Autodesk Inventor part; units mm, degrees
ref_plane "YZ Plane" through (0, 0, 0) normal (1, 0, 0) x (0, 1, 0)
ref_plane "XZ Plane" through (0, 0, 0) normal (0, 1, 0) x (-1, 0, 0)
ref_plane "XY Plane" through (0, 0, 0) normal (0, 0, 1) x (1, 0, 0)
sketch "スケッチ1" plane through (0, 0, 0) normal (0, 0, 1) x (1, 0, 0)
  line L0 (-10, 10) -> (10, 10)
  line L1 (10, 10) -> (10, -10)
  line L2 (10, -10) -> (-10, -10)
  line L3 (-10, -10) -> (-10, 10)
  line L4 (-10, 10) -> (10, -10) construction
  line L5 (10, 10) -> (-10, -10) construction
  point P0 (0, 0)
  dimension "d0" = 20
  dimension "d1" = 20
extrude "押し出し1" add sketch "スケッチ1" against normal blind 60
sketch "スケッチ2" plane through (0, 0, 0) normal (0, 0, 1) x (1, 0, 0)
  line L0 (-8, 8) -> (8, 8)
  line L1 (8, 8) -> (8, -8)
  line L2 (8, -8) -> (-8, -8)
  line L3 (-8, -8) -> (-8, 8)
  line L4 (-8, 8) -> (8, -8) construction
  line L5 (8, 8) -> (-8, -8) construction
  point P0 (0, 0)
  dimension "d4" = 16
  dimension "d5" = 16
extrude "押し出し2" cut sketch "スケッチ2" against normal blind 1
sketch "スケッチ3" plane through (0, 0, -1) normal (0, 0, 1) x (1, 0, 0)
  line L0 (-7.5, 7.5) -> (7, 7.5) construction
  line L1 (7, 7.5) -> (7, -7.5) construction
  line L2 (7, -7.5) -> (-7.5, -7.5) construction
  line L3 (-7.5, -7.5) -> (-7.5, 7.5) construction
  line L4 (-8, 8) -> (8, 8)
  line L5 (8, -8) -> (-8, -8)
  line L6 (-8, -8) -> (-8, 8)
  line L7 (8, 8) -> (8, -8)
  spline S0 degree 2 poles (-4.378, -6.0365) (-4.1155, -6.0365) (-4.1155, -5.7836) knots 0 0 0 1 1 1
  line L8 (-4.1155, -5.7836) -> (-4.1155, -1.8452)
  line L9 (-4.1155, -1.8452) -> (-5.7978, -1.8452)
  line L10 (-5.7978, -1.8452) -> (-5.7978, -3.265)
  spline S1 degree 2 poles (-5.7978, -3.265) (-5.7978, -5.5211) (-6.887, -7.1353) knots 0 0 0 1 1 1
  line L11 (-6.887, -7.1353) -> (-7.7913, -6.3574)
  spline S2 degree 2 poles (-7.7913, -6.3574) (-6.887, -4.8112) (-6.887, -2.7496) knots 0 0 0 1 1 1
  line L12 (-6.887, -2.7496) -> (-6.887, 6.6637)
  line L13 (-6.887, 6.6637) -> (-3.0263, 6.6637)
  line L14 (-3.0263, 6.6637) -> (-3.0263, -6.1045)
  spline S3 degree 2 poles (-3.0263, -6.1045) (-3.0263, -7.0673) (-3.7265, -7.0673) knots 0 0 0 1 1 1
  line L15 (-3.7265, -7.0673) -> (-4.8254, -7.0673)
  line L16 (-4.8254, -7.0673) -> (-5.0199, -6.0365)
  line L17 (-5.0199, -6.0365) -> (-4.378, -6.0365)
  line L18 (0.0758, 2.278) -> (1.8748, 2.278)
  spline S4 degree 2 poles (1.8748, 2.278) (2.1957, -4.4319) (-2.122, -7.3298) knots 0 0 0 1 1 1
  line L19 (-2.122, -7.3298) -> (-2.8902, -6.231)
  spline S5 degree 2 poles (-2.8902, -6.231) (-0.955, -5.1321) (0.0077, -2.8177) knots 0 0 0 1 1 1
  line L20 (0.0077, -2.8177) -> (-1.2176, -1.7188)
  spline S6 degree 2 poles (-1.2176, -1.7188) (-1.6649, -2.4287) (-2.1803, -2.9441) knots 0 0 0 1 1 1
  line L21 (-2.1803, -2.9441) -> (-2.8318, -1.7869)
  spline S7 degree 2 poles (-2.8318, -1.7869) (-1.2857, -0.1726) (-0.8967, 3.3088) knots 0 0 0 1 1 1
  line L22 (-0.8967, 3.3088) -> (0.2703, 3.1823)
  spline S8 degree 2 poles (0.2703, 3.1823) (0.455, 2.9878) (0.1341, 2.7934) knots 0 0 0 1 1 1
  line L23 (0.1341, 2.7934) -> (0.0758, 2.278)
  spline S9 degree 2 poles (6.3286, -2.5551) (6.3286, -3.5276) (5.6187, -3.5276) knots 0 0 0 1 1 1
  line L24 (5.6187, -3.5276) -> (4.5199, -3.5276)
  line L25 (4.5199, -3.5276) -> (4.267, -2.4968)
  line L26 (4.267, -2.4968) -> (4.9672, -2.4968)
  spline S10 degree 2 poles (4.9672, -2.4968) (5.2297, -2.4968) (5.2297, -2.2342) knots 0 0 0 1 1 1
  line L27 (5.2297, -2.2342) -> (5.2297, 1.4417)
  line L28 (5.2297, 1.4417) -> (3.6155, 1.4417)
  line L29 (3.6155, 1.4417) -> (3.6155, -5.3947)
  spline S11 degree 2 poles (3.6155, -5.3947) (3.6155, -5.842) (4.0725, -5.842) knots 0 0 0 1 1 1
  line L30 (4.0725, -5.842) -> (5.1617, -5.842)
  spline S12 degree 2 poles (5.1617, -5.842) (5.7451, -5.842) (5.8132, -5.3266) knots 0 0 0 1 1 1
  line L31 (5.8132, -5.3266) -> (6.0077, -4.1694)
  line L32 (6.0077, -4.1694) -> (7.1649, -4.4903)
  line L33 (7.1649, -4.4903) -> (6.9704, -5.7156)
  spline S13 degree 2 poles (6.9704, -5.7156) (6.7759, -6.8728) (5.8716, -6.8728) knots 0 0 0 1 1 1
  line L34 (5.8716, -6.8728) -> (3.6835, -6.8728)
  spline S14 degree 2 poles (3.6835, -6.8728) (2.5263, -6.8728) (2.5263, -5.7156) knots 0 0 0 1 1 1
  line L35 (2.5263, -5.7156) -> (2.5263, 2.4724)
  line L36 (2.5263, 2.4724) -> (6.3286, 2.4724)
  line L37 (6.3286, 2.4724) -> (6.3286, -2.5551)
  line L38 (-2.3748, 2.346) -> (-2.3748, 5.3703)
  line L39 (-2.3748, 5.3703) -> (1.4275, 5.3703)
  line L40 (1.4275, 5.3703) -> (1.4275, 7.5)
  line L41 (1.4275, 7.5) -> (2.6528, 7.5)
  spline S15 degree 2 poles (2.6528, 7.5) (3.1682, 7.4319) (2.7111, 7.111) knots 0 0 0 1 1 1
  line L42 (2.7111, 7.111) -> (2.7111, 5.3703)
  line L43 (2.7111, 5.3703) -> (6.844, 5.3703)
  line L44 (6.844, 5.3703) -> (6.844, 2.8614)
  line L45 (6.844, 2.8614) -> (5.7451, 2.8614)
  line L46 (5.7451, 2.8614) -> (5.7451, 4.3395)
  line L47 (5.7451, 4.3395) -> (-1.2857, 4.3395)
  line L48 (-1.2857, 4.3395) -> (-1.2857, 2.346)
  line L49 (-1.2857, 2.346) -> (-2.3748, 2.346)
  line L50 (-4.1155, -0.8144) -> (-4.1155, 1.957)
  line L51 (-4.1155, 1.957) -> (-5.7978, 1.957)
  line L52 (-5.7978, 1.957) -> (-5.7978, -0.8144)
  line L53 (-5.7978, -0.8144) -> (-4.1155, -0.8144)
  line L54 (-5.7978, 2.9878) -> (-4.1155, 2.9878)
  line L55 (-4.1155, 2.9878) -> (-4.1155, 5.6329)
  line L56 (-4.1155, 5.6329) -> (-5.7978, 5.6329)
  line L57 (-5.7978, 5.6329) -> (-5.7978, 2.9878)
  spline S16 degree 2 poles (-0.1187, 1.2472) (-0.3132, 0.2747) (-0.7703, -0.688) knots 0 0 0 1 1 1
  line L58 (-0.7703, -0.688) -> (0.455, -1.5243)
  spline S17 degree 2 poles (0.455, -1.5243) (0.7857, -0.2407) (0.7857, 1.2472) knots 0 0 0 1 1 1
  line L59 (0.7857, 1.2472) -> (-0.1187, 1.2472)
  point P0 (0, 0)
  dimension "d8" = 0.5
  dimension "d9" = 0.5
  dimension "d10" = 0.5
  dimension "d11" = 1
extrude "押し出し3" add sketch "スケッチ3" along normal blind 1 contours S0 L8 L9 L10 S1 L11 S2 L12 L13 L14 S3 L15 L16 L17 | L18 S4 L19 S5 L20 S6 L21 S7 L22 S8 L23 | S9 L24 L25 L26 S10 L27 L28 L29 S11 L30 S12 L31 L32 L33 S13 L34 S14 L35 L36 L37 | L38 L39 L40 L41 S15 L42 L43 L44 L45 L46 L47 L48 L49
properties part number "ハンコ"
Here's how the part is built. I have some questions about the finished solid (model axes, mm). Coordinates: 2 decimals unless noted, no trailing zeros.
Item 1: I need wall thicknesses on probe 1 along Z at (x, y) = (4, 6). Which ranges of the line are inside material? Lowest first, please.
Response values:
probe 1: z = -60 to -1
Item 2: Thinking about a two-plate mould opening in X: for faces 1 (the face through (-4.9, 1.957, -0.5)), 2 (the face through (0, -2, 0)), 3 (the face through (6.844, 4.1, -0.5)), which applies, pulls with the +X half, pulls with the -X half, needs draft (parallel to the pull), parting line crosses it, or undercut?
Response values:
face 1: undercut
face 2: needs draft
face 3: undercut
Item 3: I'm going to push a flat-ended pin straight in: pin 1 Ø1.3 at (x, y) = (-5, 4.5) entering from +Z. Where does the tip first touch, or does it pass through?
Response values:
pin 1: stops at z = -1
